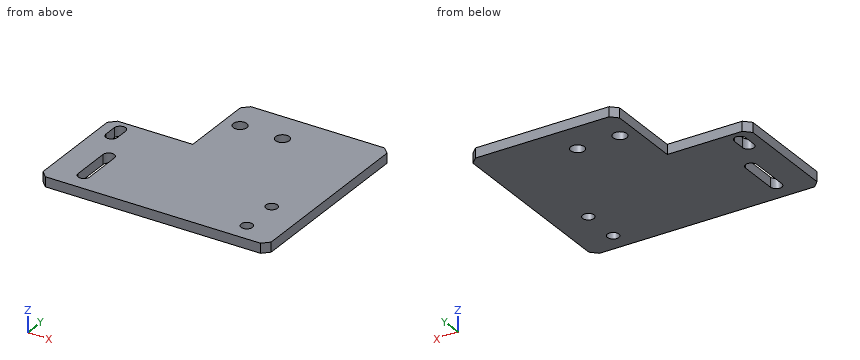
from build123d import *

# Parameters (mm, degrees)
SKETCH1_R           = 1.75
SKETCH1_R_2         = 2.096313729
BOSS_EXTRUDE1_DEPTH = 3
CHAMFER1_SIZE       = 2


with BuildPart() as part:
    # Sketch1 → Boss-Extrude1 (new body)
    with BuildSketch(Plane.XY):
        Polygon((-11.830357143, 26.84375), (33.169642857, 26.84375), (33.169642857, -33.15625), (-36.830357143, -33.15625), (-36.830357143, 1.84375), (-11.830357143, 1.84375), align=None)
        with Locations((23.169642857, -15.15625)):
            Circle(SKETCH1_R, mode=Mode.SUBTRACT)
        with Locations((23.169642857, -27.15625)):
            Circle(SKETCH1_R, mode=Mode.SUBTRACT)
        with Locations((6.169642857, 16.84375)):
            Circle(SKETCH1_R_2, mode=Mode.SUBTRACT)
        with Locations((-6.830357143, 16.84375)):
            Circle(SKETCH1_R_2, mode=Mode.SUBTRACT)
        with BuildLine():
            Line((-25.080357143, -15.15625), (-25.080357143, -27.15625))
            ThreePointArc((-25.080357143, -27.15625), (-26.830357143, -28.90625), (-28.580357143, -27.15625))
            Line((-28.580357143, -27.15625), (-28.580357143, -15.15625))
            ThreePointArc((-28.580357143, -15.15625), (-26.830357143, -13.40625), (-25.080357143, -15.15625))
        make_face(mode=Mode.SUBTRACT)
        with BuildLine():
            Line((-33.75, -1.558035714), (-33.75, -5.558035714))
            ThreePointArc((-33.75, -5.558035714), (-32, -7.308035714), (-30.25, -5.558035714))
            Line((-30.25, -5.558035714), (-30.25, -1.558035714))
            ThreePointArc((-30.25, -1.558035714), (-32, 0.191964286), (-33.75, -1.558035714))
        make_face(mode=Mode.SUBTRACT)
    extrude(amount=BOSS_EXTRUDE1_DEPTH)

    # Chamfer1
    chamfer1_edges = [part.edges().sort_by_distance(p)[0] for p in [
        (-11.830357143, 26.84375, 1.5),
        (33.169642857, 26.84375, 1.5),
        (33.169642857, -33.15625, 1.5),
        (-36.830357143, -33.15625, 1.5),
        (-36.830357143, 1.84375, 1.5),
    ]]
    chamfer(chamfer1_edges, length=CHAMFER1_SIZE)


solid = part.part
Model file for the job. Use its own axes, mm. Give positions to 0.01 mm unless a question says otherwise; leave off trailing zeros. Loops run counter-clockwise (first coordinate to the right, second up) from the corner with the lowest first, then second, coordinate; pieces in that order, holes last. Notation, with made-up numbers: (-1, 8.5) - (9, 8.5) arc R26 ccw to (9, 35.5) - close; hole circle Ø3 at (4.5, 28). An arc over 180 degrees is marked (long way). Use one line per item in the form item = value.
(1) Cut at D-D (y = 21). Give the cut face in (x, z).
Determined:
outline = (-11.83, 0) - (33.17, 0) - (33.17, 3) - (-11.83, 3) - close
(2) Drop flat-ended pins along their axis: P1, Ø3, axis at x = 23.17, y = -27.16, coming from the +Z side; P2, Ø1.5, axis at y = 12.5, z = 1.5, coming from the -X side. Give the stop position or say it passes through.
Determined:
P1 = through
P2 = -11.83
(3) Cut at C-C (z = 1.8). Give the cut face in (x, y).
Determined:
outline = (-36.83, -31.16) - (-34.83, -33.16) - (31.17, -33.16) - (33.17, -31.16) - (33.17, 24.84) - (31.17, 26.84) - (-9.83, 26.84) - (-11.83, 24.84) - (-11.83, 1.84) - (-34.83, 1.84) - (-36.83, -0.16) - close; hole (-33.75, -5.56) arc R1.75 ccw to (-30.25, -5.56) - (-30.25, -1.56) arc R1.75 ccw to (-33.75, -1.56) - close; hole (-28.58, -27.16) arc R1.75 ccw to (-25.08, -27.16) - (-25.08, -15.16) arc R1.75 ccw to (-28.58, -15.16) - close; hole circle Ø4.19 at (-6.83, 16.84); hole circle Ø4.19 at (6.17, 16.84); hole circle Ø3.5 at (23.17, -27.16); hole circle Ø3.5 at (23.17, -15.16)
(4) Cut at A-A (x = -32). Give the cut face in (y, z).
Determined:
outline = (-33.16, 0) - (-7.31, 0) - (-7.31, 3) - (-33.16, 3) - close; (0.19, 0) - (1.84, 0) - (1.84, 3) - (0.19, 3) - close
(5) Cut at B-B (x = 24). Give the cut face in (y, z), then the cut area to 3 significant figures.
Determined:
outline = (-33.16, 0) - (-28.7, 0) - (-28.7, 3) - (-33.16, 3) - close; (-25.62, 0) - (-16.7, 0) - (-16.7, 3) - (-25.62, 3) - close; (-13.62, 0) - (26.84, 0) - (26.84, 3) - (-13.62, 3) - close
area = 162 mm^2
(6) Drill centre lines: L1, parallel to X at y = -2.5, z = 2.1; L2, parallel to X at y = -18, z = 0.3; L3, parallel to Y at x = -16, z = 0.2. Where is each one in solid material? Low to high.
Determined:
L1 = -36.83 to -33.75, -30.25 to 33.17
L2 = -36.83 to -28.58, -25.08 to 33.17
L3 = -33.16 to 1.84
